from build123d import *

# Parameters (mm, degrees)
SKIZZE1_R                        = 50
SKIZZE1_R_2                      = 40
AUFSATZ_LINEAR_AUSTRAGEN1_DEPTH  = 9
F_3_1_3_1_DURCHMESSER_BOHRUNG1_D = 3.1
KREISMUSTER1_COUNT               = 7
SKIZZE4_R                        = 3.1
SCHNITT_LINEAR_AUSTRAGEN1_DEPTH  = 3.3
KREISMUSTER2_COUNT               = 7


with BuildPart() as part:
    # Skizze1 → Aufsatz-Linear austragen1 (new body)
    with BuildSketch(Plane.XY):
        Circle(SKIZZE1_R)
        Circle(SKIZZE1_R_2, mode=Mode.SUBTRACT)
    extrude(amount=AUFSATZ_LINEAR_AUSTRAGEN1_DEPTH)

    # Ø3.1 (3.1) Durchmesser Bohrung1 (through all)
    with Locations(Plane.XY.offset(9)):
        with Locations((0, 46)):
            f_3_1_3_1_durchmesser_bohrung1 = Hole(F_3_1_3_1_DURCHMESSER_BOHRUNG1_D / 2)

    # Kreismuster1: Ø3.1 (3.1) Durchmesser Bohrung1 ×7 about axis
    kreismuster1_axis = Axis((0, 0, 0), (0, 0, 1))
    for i in range(1, KREISMUSTER1_COUNT):
        add(f_3_1_3_1_durchmesser_bohrung1.rotate(kreismuster1_axis, i * 360 / KREISMUSTER1_COUNT), mode=Mode.SUBTRACT)

    # Skizze4 → Schnitt-Linear austragen1 (cut)
    with BuildSketch(Plane.XY):
        with Locations((0, 46)):
            Circle(SKIZZE4_R)
    schnitt_linear_austragen1 = extrude(amount=SCHNITT_LINEAR_AUSTRAGEN1_DEPTH, mode=Mode.SUBTRACT)

    # Kreismuster2: Schnitt-Linear austragen1 ×7 about axis
    kreismuster2_axis = Axis((0, 0, 0), (0, 0, 1))
    for i in range(1, KREISMUSTER2_COUNT):
        add(schnitt_linear_austragen1.rotate(kreismuster2_axis, i * 360 / KREISMUSTER2_COUNT), mode=Mode.SUBTRACT)


solid = part.part
Can you work these out from the model? Positions are in its coordinate system, mm. A direction names the side the tool comes from. Round coordinates to 2 decimals unless told otherwise and drop trailing zeros. Loops run counter-clockwise (first coordinate to the right, second up) from the corner with the lowest first, then second, coordinate; pieces in that order, holes last. Notation, with made-up numbers: (59.5, -15.75) - (78.5, -15.75) arc R21 ccw to (78.5, 16.25) - close; hole circle Ø10 at (53.5, 73.5). An arc over 180 degrees is marked (long way). Use CSV: the item, a comma, the result in double quotes. Start each with the question number.
1) For faces 1 (the flat face through (-38, 29, 3.3)), 2 (the cylindrical face through (0.336, 44.487, 6.11)), which set-ups out of +Z, -Z, +X, -X, +Y, -Y let a thin tool reach every point of the face, with its end or its side?
2) Please list where these lines run through material, in increasing order: probe 1 along Y at (x, z) = (0, 6.7); probe 2 along Y at (x, z) = (0, 0.7); probe 3 along Y at (x, z) = (-16.5, 4.25). Write a range as [from, to].
3) If we section it at B-B on x = 0: Write out the boundary of the cut face in (y, z).
4) If we section it at A-A on y = 0: Write out the boundary of the cut face in (x, z), plus the area to 3 significant figures.
5) If we section it at C-C on z = 7.75: Count the separate pieces of the cut face and the enclosed holes in it, plus the area to 3 significant figures.
6) We'd pull the mould along X, two halves only. Please class faces 3 (the flat face through (43, -11, 3.3)), 4 (the flat face through (-4, -41, 9)): released by +X, released by -X, zero draft, split by the parting line, or undercut.
7) If we section it at D-D on x = 25.5: Write out the boundary of the cut face in (y, z).
8) For pin 1 Ø5 at (x, y) = (-44.85, -10.24) entering from -Z; pin 2 Ø4 at (x, z) = (26, 4.5) entering from +Y; pin 3 Ø5 at (x, z) = (-35, 2.5) entering from +Y, each with a flat end and sliding along its axis, tell me the tip position at first contact or that it passes through.
Geometry results:
1,face 1,"-Z"
1,face 2,"+Z, -Z"
2,probe 1,"y = [-50, -40], [40, 44.45], [47.55, 50]"
2,probe 2,"y = [-50, -40], [40, 42.9], [49.1, 50]"
2,probe 3,"y = [-47.2, -36.44], [36.44, 47.2]"
3,outline,"(-50, 0) - (-40, 0) - (-40, 9) - (-50, 9) - close; (40, 0) - (42.9, 0) - (42.9, 3.3) - (44.45, 3.3) - (44.45, 9) - (40, 9) - close; (47.55, 3.3) - (49.1, 3.3) - (49.1, 0) - (50, 0) - (50, 9) - (47.55, 9) - close"
4,outline,"(-50, 0) - (-40, 0) - (-40, 9) - (-50, 9) - close; (40, 0) - (50, 0) - (50, 9) - (40, 9) - close"
4,area,"180 mm2"
5,separate pieces,"1"
5,enclosed holes,"8"
5,area,"2,770 mm2"
6,face 3,"undercut"
6,face 4,"zero draft"
7,outline,"(-43.01, 0) - (-30.82, 0) - (-30.82, 9) - (-43.01, 9) - close; (30.82, 0) - (43.01, 0) - (43.01, 9) - (30.82, 9) - close"
8,pin 1,"stops at z = 3.3"
8,pin 2,"stops at y = 43.86"
8,pin 3,"stops at y = 38"
